Work out the finished part from the listing and answer in its coordinate system (mm). A direction names the side the tool comes from. Round coordinates to 2 decimals unless told otherwise and drop trailing zeros. Order: outer loops, then holes, each group sorted by start corner. A loop starts at its lowest first (then second) coordinate and runs counter-clockwise, first axis right, second up. Notation, with made-up numbers: (70, 13.25) - (88, 13.25) arc R13 cw to (88, 22.25) - close; hole circle Ø8 at (86, -35.5). An arc over 180 degrees is marked (long way). Put each result on its own line as item: value.
```python
from build123d import *

# Parameters (mm, degrees)
ESQUISSE1_R          = 2
BOSS_EXTRU_1_DEPTH   = 50
BOSS_EXTRU_1_2_DEPTH = 50
BOSS_EXTRU_1_3_DEPTH = 50
BOSS_EXTRU_1_4_DEPTH = 50
ESQUISSE2_W          = 226.6
ESQUISSE2_H          = 69.9
BOSS_EXTRU_2_DEPTH   = 5


with BuildPart() as part:
    # Esquisse1 → Boss.-Extru.1 (new body)
    with BuildSketch(Plane(origin=(0, 0, 0), x_dir=(1, 0, 0), z_dir=(0, 1, 0))):
        Polygon((-113.3, -27.45), (-113.3, -19.95), (-98.3, -19.95), (-98.3, -34.95), (-113.3, -34.95), align=None)
        with Locations(Location((-105.8, -27.45, 0), (0, 0, 270))):
            Circle(ESQUISSE1_R, mode=Mode.SUBTRACT)
    extrude(amount=BOSS_EXTRU_1_DEPTH)



with BuildPart() as body_2:
    # Esquisse1 → Boss.-Extru.1 2 (new body)
    with BuildSketch(Plane(origin=(0, 0, 0), x_dir=(1, 0, 0), z_dir=(0, 1, 0))):
        Polygon((-113.3, -74.85), (-113.3, -82.35), (-113.3, -89.85), (-98.3, -89.85), (-98.3, -74.85), align=None)
        with Locations(Location((-105.8, -82.35, 0), (0, 0, 90))):
            Circle(ESQUISSE1_R, mode=Mode.SUBTRACT)
    extrude(amount=BOSS_EXTRU_1_2_DEPTH)


with BuildPart() as body_3:
    # Esquisse1 → Boss.-Extru.1 3 (new body)
    with BuildSketch(Plane(origin=(0, 0, 0), x_dir=(1, 0, 0), z_dir=(0, 1, 0))):
        Polygon((98.3, -74.85), (113.3, -74.85), (113.3, -82.35), (113.3, -89.85), (98.3, -89.85), align=None)
        with Locations(Location((105.8, -82.35, 0), (0, 0, 270))):
            Circle(ESQUISSE1_R, mode=Mode.SUBTRACT)
    extrude(amount=BOSS_EXTRU_1_3_DEPTH)


with BuildPart() as body_4:
    # Esquisse1 → Boss.-Extru.1 4 (new body)
    with BuildSketch(Plane(origin=(0, 0, 0), x_dir=(1, 0, 0), z_dir=(0, 1, 0))):
        Polygon((113.3, -34.95), (113.3, -27.45), (113.3, -19.95), (98.3, -19.95), (98.3, -34.95), align=None)
        with Locations(Location((105.8, -27.45, 0), (0, 0, 90))):
            Circle(ESQUISSE1_R, mode=Mode.SUBTRACT)
    extrude(amount=BOSS_EXTRU_1_4_DEPTH)


with BuildPart() as part_1:
    add(part.part)

    add(body_2.part)  # Boss.-Extru.2 merges body 2

    add(body_3.part)  # Boss.-Extru.2 merges body 3

    add(body_4.part)  # Boss.-Extru.2 merges body 4
    # Esquisse2 → Boss.-Extru.2 (add)
    with BuildSketch(Plane(origin=(0, 50, 0), x_dir=(1, 0, 0), z_dir=(0, 1, 0))):
        with Locations((0, -54.9)):
            Rectangle(ESQUISSE2_W, ESQUISSE2_H)
    extrude(amount=BOSS_EXTRU_2_DEPTH)


solid = part_1.part
```
1) Given pin 1 Ø3 at (x, z) = (105.8, 82.35) entering from -Y, flat-ended and moving along its own axis, determine where the tip first touches the part or whether it passes through.
Findings below:
pin 1: stops at y = 50
2) For faces 4 (the flat face through (-106, 25, 74.85)), 5 (the flat face through (-108, 0, 81)), 6 (the cylindrical face through (103.817, 24.65, 27.71)), 7 (the flat face through (-98.3, 25, 82)), determine the directions among +Z, -Z, +X, -X, +Y, -Y from which every point of the face is accessible in a straight line to the end or side of a thin tool.
Findings below:
face 4: +X, -X, -Y
face 5: +Z, -Z, +X, -X, -Y
face 6: -Y
face 7: +Z, -Z, -Y
3) Straight lines are drawn through the part: L1, parallel to X at y = 15.5, z = 27.45; L2, parallel to Z at x = 105, y = 38; L3, parallel to Y at x = -10, z = 25.5. For each, find the intervals that lie inside material, in ascending order. Write a range as from..to.
Findings below:
L1: x = -113.3..-107.8, -103.8..-98.3, 98.3..103.8, 107.8..113.3
L2: z = 19.95..25.62, 29.28..34.95, 74.85..80.52, 84.18..89.85
L3: y = 50..55
4) A cutting plane is placed at B-B on z = 27.45. Write down the section's boundary in (x, y), then the cut area to 3 significant figures.
Findings below:
outline: (-113.3, 0) - (-107.8, 0) - (-107.8, 50) - (-103.8, 50) - (-103.8, 0) - (-98.3, 0) - (-98.3, 50) - (98.3, 50) - (98.3, 0) - (103.8, 0) - (103.8, 50) - (107.8, 50) - (107.8, 0) - (113.3, 0) - (113.3, 55) - (-113.3, 55) - close
area: 2,230 mm2
5) A cutting plane is placed at C-C on x = 105.8. Write down the section's boundary in (y, z).
Findings below:
outline: (0, 19.95) - (55, 19.95) - (55, 89.85) - (0, 89.85) - (0, 84.35) - (50, 84.35) - (50, 80.35) - (0, 80.35) - (0, 74.85) - (50, 74.85) - (50, 34.95) - (0, 34.95) - (0, 29.45) - (50, 29.45) - (50, 25.45) - (0, 25.45) - close
6) A cutting plane is placed at A-A on y = 22. Write down the section's boundary in (x, z), then the cut area to 3 significant figures.
Findings below:
outline: (-113.3, 19.95) - (-98.3, 19.95) - (-98.3, 34.95) - (-113.3, 34.95) - close; (-113.3, 74.85) - (-98.3, 74.85) - (-98.3, 89.85) - (-113.3, 89.85) - close; (98.3, 19.95) - (113.3, 19.95) - (113.3, 34.95) - (98.3, 34.95) - close; (98.3, 74.85) - (113.3, 74.85) - (113.3, 89.85) - (98.3, 89.85) - close; hole circle Ø4 at (-105.8, 27.45); hole circle Ø4 at (-105.8, 82.35); hole circle Ø4 at (105.8, 27.45); hole circle Ø4 at (105.8, 82.35)
area: 850 mm2
7) For a pull along Z with two mould halves and no side action, classify faces 1 (the flat face through (-104, 0, 29)), 2 (the flat face through (-106, 50, 82)), 3 (the flat face through (-1, 52, 19.95)) as pulls with the +Z half, pulls with the -Z half, needs draft (parallel to the pull), parting line crosses it, or undercut.
Findings below:
face 1: needs draft
face 2: undercut
face 3: pulls with the -Z half
8) A cutting plane is placed at D-D on z = 64. Write down the section's boundary in (x, y), then the cut area to 3 significant figures.
Findings below:
outline: (-113.3, 50) - (113.3, 50) - (113.3, 55) - (-113.3, 55) - close
area: 1,130 mm2
